from build123d import *

# Parameters (mm, degrees)
CUT_EXTRUDE1_DEPTH = 1.5875


with BuildPart() as part:
    # Sketch1 → Revolve1 (revolve)
    with BuildSketch(Plane.XY, mode=Mode.PRIVATE) as revolve1_sk:
        Polygon((-69.85, 0), (-69.85, 3.175), (-58.7375, 3.175), (-58.7375, 6.35), (-50.8, 6.35), (-50.8, 5.9436), (-49.8094, 5.9436), (-49.8094, 6.35), (0, 6.35), (0, 0), align=None)
    revolve(revolve1_sk.sketch.rotate(Axis((0, 0, 0), (-1, 0, 0)), 90), axis=Axis((0, 0, 0), (-1, 0, 0)))

    # Sketch2 → Cut-Extrude1 (cut)
    with BuildSketch(Plane(origin=(0, 6.35, 0), x_dir=(-1, 0, 0), z_dir=(0, 1, 0))):
        with BuildLine():
            Line((19.05, 1.5875), (0, 1.5875))
            Line((0, 1.5875), (0, -1.5875))
            Line((0, -1.5875), (19.05, -1.5875))
            ThreePointArc((19.05, -1.5875), (20.6375, 0), (19.05, 1.5875))
        make_face()
    extrude(amount=-CUT_EXTRUDE1_DEPTH, mode=Mode.SUBTRACT)


solid = part.part
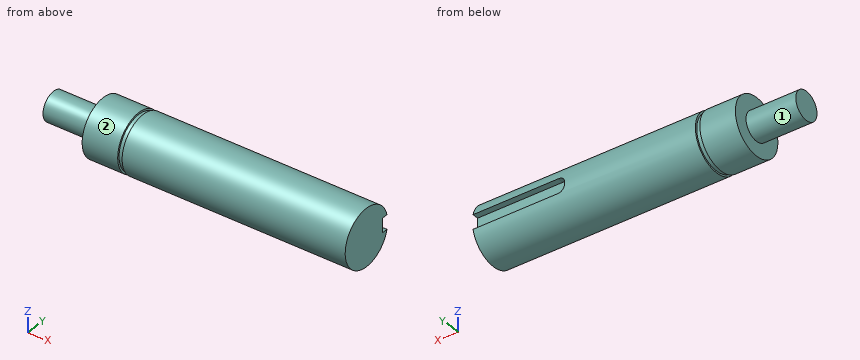
Verification items for the finished model (mm, model axes). Face numbers are marked on the shaded views. A direction names the side the tool comes from. Give positions to 0.01 mm unless a question says otherwise; leave off trailing zeros. Loops run counter-clockwise (first coordinate to the right, second up) from the corner with the lowest first, then second, coordinate; pieces in that order, holes last. Notation, with made-up numbers: (41.5, -26) - (58.5, -26) arc R22 cw to (58.5, 8) - close; hole circle Ø10 at (-28.5, -19.5). An arc over 180 degrees is marked (long way). Write item = value, one per line. Start each with the question number.
Q1. Tool access check on the marked faces 1 and 2. Record the directions out of +Z, -Z, +X, -X, +Y, -Y that give a thin tool (end or side, any length) a straight path to the whole face; none if there is none.
Q2. Cross-section at D-D, the plane x = -29. Enter the section's corners in (y, z), and give its area (3 significant figures).
Q3. Depth check by flat-ended pin: P1, Ø1.6, axis at x = -11.5, z = 0.5, coming from the +Y side; P2, Ø3, axis at x = -47.5, z = 2, coming from the -Y side; P3, Ø0.7, axis at x = -7.5, y = 5, coming from the +Z side. Enter the tip coordinate at first touch or a pass-through.
Q4. Cross-section at C-C, the plane x = -61.5. Enter the section's corners in (y, z) (3 decimals).
Q5. Thickness scan on line 1 (Z direction, x = -13.5, y = 2.25); line 2 (Z direction, x = -2.5, y = -0.25); line 3 (X direction, y = -4.25, z = -0.75). Record the ranges inside material, lowest first.
Answer key:
q1.face_1 = -X
q1.face_2 = +X, -X
q2.outline = circle Ø12.7 at (0, 0)
q2.area = 127 mm^2
q3.P1 = 4.76
q3.P2 = -6.33
q3.P3 = 4.32
q4.outline = circle Ø6.35 at (0, 0)
q5.line_1 = -5.94 to 5.94
q5.line_2 = -6.35 to 6.35
q5.line_3 = -58.74 to 0
